```python
from build123d import *

# Parameters (mm, degrees)
SKETCH1_W                       = 18.4
SKETCH1_H                       = 12.5
BOSS_EXTRUDE1_DEPTH             = 55.5
SKETCH2_W                       = 2.5
SKETCH2_H                       = 1
CUT_EXTRUDE1_DEPTH              = 56.5
M2X0_4_TAPPED_HOLE1_D           = 1.6
M2X0_4_TAPPED_HOLE1_DEPTH       = 6.5
M2X0_4_TAPPED_HOLE1_CBORE_D     = 2
M2X0_4_TAPPED_HOLE1_CBORE_DEPTH = 4.5
M2X0_4_TAPPED_HOLE1_TIP         = 0.480688495
CBORE_FOR_M2_SHCS1_D            = 2.4
CBORE_FOR_M2_SHCS1_CBORE_D      = 4.4
CBORE_FOR_M2_SHCS1_CBORE_DEPTH  = 10.9
CHAMFER1_SIZE                   = 10
CHAMFER1_SIZE2                  = 4.663076582
CHAMFER2_SIZE                   = 10
CHAMFER2_SIZE2                  = 4.663076582
SKETCH7_W                       = 55.5
SKETCH7_H                       = 7.5
CUT_EXTRUDE2_DEPTH              = 9
FILLET2_R                       = 2.5


with BuildPart() as part:
    # Sketch1 → Boss-Extrude1 (new body)
    with BuildSketch(Plane.XY):
        with Locations((-9.2, 6.25)):
            Rectangle(SKETCH1_W, SKETCH1_H)
    extrude(amount=BOSS_EXTRUDE1_DEPTH)

    # Sketch2 → Cut-Extrude1 (cut, through all)
    with BuildSketch(Plane.XY.offset(55.5)):
        with Locations((-2.75, 0.5)):
            Rectangle(SKETCH2_W, SKETCH2_H)
    extrude(amount=-CUT_EXTRUDE1_DEPTH, mode=Mode.SUBTRACT)

    # M2x0.4 Tapped Hole1
    with Locations(Plane.ZY.offset(18.4)):
        with Locations((51.75, 3), (27.75, 3), (3.75, 3)):
            CounterBoreHole(M2X0_4_TAPPED_HOLE1_D / 2, M2X0_4_TAPPED_HOLE1_CBORE_D / 2, M2X0_4_TAPPED_HOLE1_CBORE_DEPTH, depth=M2X0_4_TAPPED_HOLE1_DEPTH)
            with Locations((0, 0, -(M2X0_4_TAPPED_HOLE1_DEPTH + M2X0_4_TAPPED_HOLE1_TIP / 2))):  # 118° drill point
                Cone(0, M2X0_4_TAPPED_HOLE1_D / 2, M2X0_4_TAPPED_HOLE1_TIP, mode=Mode.SUBTRACT)

    # CBORE for M2 SHCS1 (through all)
    with Locations(Plane.ZY.offset(18.4)):
        with Locations((47.75, 10), (7.75, 10)):
            CounterBoreHole(CBORE_FOR_M2_SHCS1_D / 2, CBORE_FOR_M2_SHCS1_CBORE_D / 2, CBORE_FOR_M2_SHCS1_CBORE_DEPTH)

    # Chamfer1
    chamfer1_edges = [part.edges().sort_by_distance(p)[0] for p in [
        (-9.2, 12.5, 0),
    ]]
    chamfer1_side = [part.faces().sort_by_distance(p)[0] for p in [
        (-9.270879121, 6.313186813, 0),
    ]]
    chamfer(chamfer1_edges, length=CHAMFER1_SIZE, length2=CHAMFER1_SIZE2, reference=chamfer1_side[0])

    # Chamfer2
    chamfer2_edges = [part.edges().sort_by_distance(p)[0] for p in [
        (-9.2, 12.5, 55.5),
    ]]
    chamfer2_side = [part.faces().sort_by_distance(p)[0] for p in [
        (-9.270879121, 6.313186813, 55.5),
    ]]
    chamfer(chamfer2_edges, length=CHAMFER2_SIZE, length2=CHAMFER2_SIZE2, reference=chamfer2_side[0])

    # Sketch7 → Cut-Extrude2 (cut)
    with BuildSketch(Plane.ZY.offset(18.4)):
        with Locations((27.75, 8.75)):
            Rectangle(SKETCH7_W, SKETCH7_H)
    extrude(amount=-CUT_EXTRUDE2_DEPTH, mode=Mode.SUBTRACT)

    # Fillet2
    fillet2_edges = [part.edges().sort_by_distance(p)[0] for p in [
        (-9.4, 5, 27.75),
    ]]
    fillet(fillet2_edges, radius=FILLET2_R)


solid = part.part
```
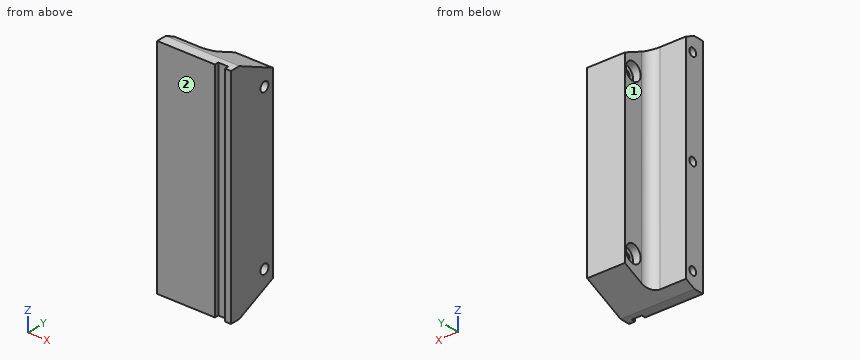
Geometry: final body of the model. Coordinates: model frame, mm. Face numbers are marked on the shaded views. A direction names the side the tool comes from. Coordinates: 2 decimals unless noted, no trailing zeros. Order: outer loops, then holes, each group sorted by start corner. A loop starts at its lowest first (then second) coordinate and runs counter-clockwise, first axis right, second up. Notation, with made-up numbers: (53.5, 20.25) -> (62.5, 20.25) arc R23 ccw to (62.5, 34.25) -> close; hole circle Ø2 at (88.25, -25). An arc over 180 degrees is marked (long way). Write item = value, one per line.
(1) Cut plane A-A on z = 47.75. Return loops of the section in (x, y).
Solved:
outline = (-18.4, 0) -> (-4, 0) -> (-4, 1) -> (-1.5, 1) -> (-1.5, 0) -> (0, 0) -> (0, 8.8) -> (-7.5, 8.8) -> (-7.5, 7.8) -> (-9.4, 7.8) -> (-9.4, 7.5) arc R2.5 cw to (-11.9, 5) -> (-18.4, 5) -> close; (-9.4, 12.2) -> (-7.5, 12.2) -> (-7.5, 11.2) -> (0, 11.2) -> (0, 12.5) -> (-9.4, 12.5) -> close
(2) Cut plane C-C on x = -6.5. Return loops of the section in (y, z), plus the area to 3 significant figures.
Solved:
outline = (0, 0) -> (2.5, 0) -> (12.5, 4.66) -> (12.5, 50.84) -> (2.5, 55.5) -> (0, 55.5) -> close; hole circle Ø2.4 at (10, 7.75); hole circle Ø2.4 at (10, 47.75)
area = 638 mm²
(3) Cut plane B-B on y = 10. Return loops of the section in (x, z), plus the area to 3 significant figures.
Solved:
outline = (-9.4, 3.5) -> (0, 3.5) -> (0, 6.55) -> (-7.5, 6.55) -> (-7.5, 5.55) -> (-9.4, 5.55) -> close; (-9.4, 9.95) -> (-7.5, 9.95) -> (-7.5, 8.95) -> (0, 8.95) -> (0, 46.55) -> (-7.5, 46.55) -> (-7.5, 45.55) -> (-9.4, 45.55) -> close; (-9.4, 49.95) -> (-7.5, 49.95) -> (-7.5, 48.95) -> (0, 48.95) -> (0, 52) -> (-9.4, 52) -> close
area = 403 mm²
(4) Pin query (flat end, axial travel): pin 1 Ø2 at (y, z) = (9.5, 47.5) entering from -X; pin 2 Ø10 at (x, z) = (-12.5, 14.5) entering from +Y; pin 3 Ø1 at (y, z) = (3, 3.5) entering from -X; pin 4 Ø2 at (x, z) = (-16, 25) entering from +Y. Return the tip coordinate at first contact, or that it passes through.
Solved:
pin_1 = -7.5
pin_2 = 12.5
pin_3 = -11.87
pin_4 = 5
(5) Access query for the marked faces 1 and 2. Directions: +Z, -Z, +X, -X, +Y, -Y. A direction counts if a zero-diameter tool reaches every point of the face in a straight line with its end or side. Return the directions, or none.
Solved:
face_1 = +Z, -Z, -X, +Y
face_2 = +Z, -Z, +X, -X, -Y
(6) Cut plane D-D on z = 37. Return loops of the section in (x, y).
Solved:
outline = (-18.4, 0) -> (-4, 0) -> (-4, 1) -> (-1.5, 1) -> (-1.5, 0) -> (0, 0) -> (0, 12.5) -> (-9.4, 12.5) -> (-9.4, 7.5) arc R2.5 cw to (-11.9, 5) -> (-18.4, 5) -> close
(7) Line query: line 1 (Y direction, x = -17.25, z = 51.75); line 2 (Z direction, x = -13, y = 3); line 3 (Z direction, x = -7.25, y = 9.75). Output: solid intervals per line, ascending.
Solved:
line_1 = 0 to 2, 4 to 5
line_2 = 0.23 to 2.95, 4.55 to 26.95, 28.55 to 50.95, 52.55 to 55.27
line_3 = 3.38 to 6.58, 8.92 to 46.58, 48.92 to 52.12
